Part print with two shaded views. Sizes in mm from the minimum x, y, z corner. Coordinates: 2 decimals unless noted, no trailing zeros. Loops run counter-clockwise (first coordinate to the right, second up) from the corner with the lowest first, then second, coordinate; pieces in that order, holes last. Notation, with made-up numbers: (28.5, 36.5) - (35.5, 36.5) arc R10 cw to (35.5, 52.5) - close; hole circle Ø3 at (12, 7.5). An arc over 180 degrees is marked (long way). Answer as CSV lines item,"result".
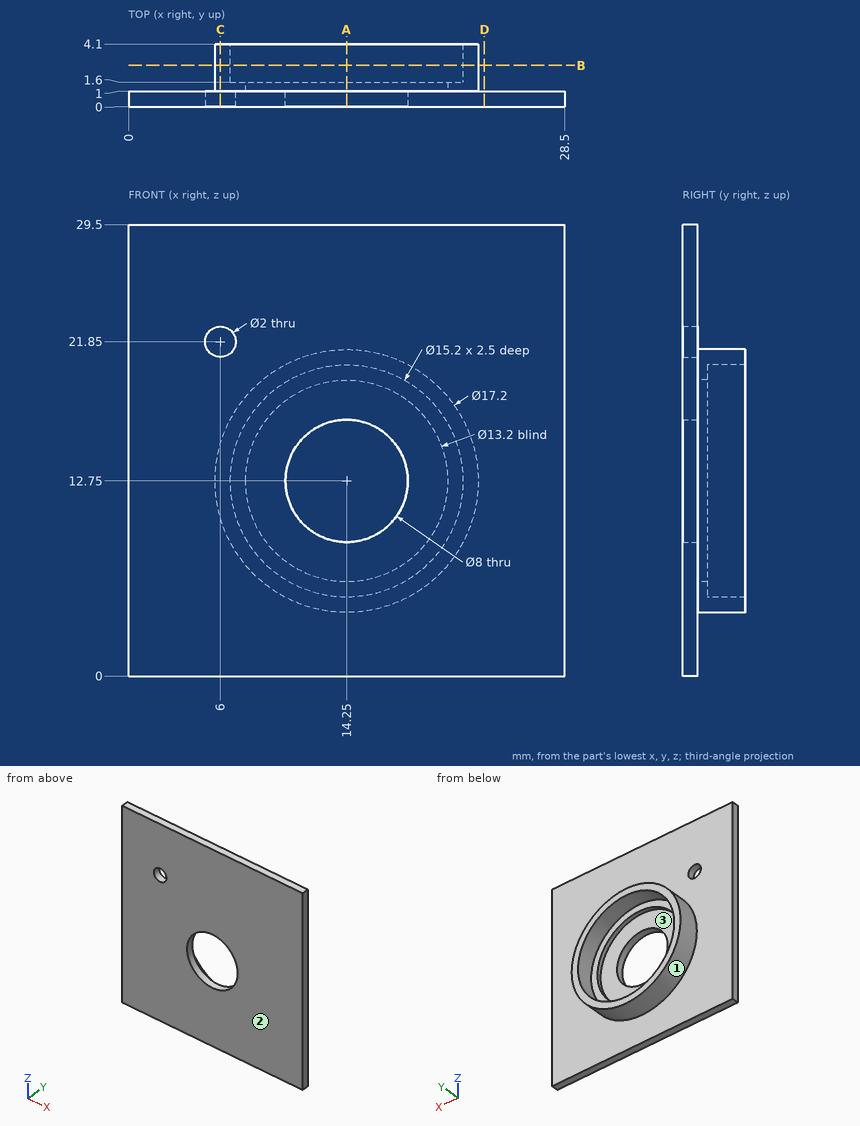
Q1. Saw through at C-C (x = 6). Give the cut face in (y, z).
Results:
outline,"(0, 0) - (1, 0) - (1, 10.32) - (4.1, 10.32) - (4.1, 15.18) - (1, 15.18) - (1, 20.85) - (0, 20.85) - close; (0, 22.85) - (1, 22.85) - (1, 29.5) - (0, 29.5) - close"
Q2. Wall check: L1, parallel to X at y = 0.7, z = 21.85; L2, parallel to Z at x = 14.25, y = 1.25; L3, parallel to Z at x = 6, y = 0.3. Give the ranges that are in metal, low to high.
Results:
L1,"x = 0 to 5, 7 to 28.5"
L2,"z = 4.15 to 6.15, 19.35 to 21.35"
L3,"z = 0 to 20.85, 22.85 to 29.5"
Q3. Two-plate mould, pull along Z, no slides. Class the marked faces 1, 2 and 3: released by +Z, released by -Z, zero draft, split by the parting line, or undercut.
Results:
face 1,"split by the parting line"
face 2,"zero draft"
face 3,"undercut"
Q4. Saw through at A-A (x = 14.25). Give the cut face in (y, z), then the cut area to 3 significant figures.
Results:
outline,"(0, 0) - (1, 0) - (1, 4.15) - (4.1, 4.15) - (4.1, 5.15) - (1.6, 5.15) - (1.6, 6.15) - (1, 6.15) - (1, 8.75) - (0, 8.75) - close; (0, 16.75) - (1, 16.75) - (1, 19.35) - (1.6, 19.35) - (1.6, 20.35) - (4.1, 20.35) - (4.1, 21.35) - (1, 21.35) - (1, 29.5) - (0, 29.5) - close"
area,"28.9 mm^2"
Q5. Flat gauge pins, fed straight in: pin 1 (8 mm diameter, centred on x = 6, z = 26, fed in from +Y); pin 2 (2 mm diameter, centred on y = 2.5, z = 19.5, fed in from +X); pin 3 (1.5 mm diameter, centred on y = 2.5, z = 6, fed in from -X). Where does each tip first touch, or does it go through?
Results:
pin 1,"stops at y = 1"
pin 2,"stops at x = 20.65"
pin 3,"stops at x = 8.09"
Q6. Saw through at D-D (x = 23.25). Give the cut face in (y, z), then the cut area to 3 significant figures.
Results:
outline,"(0, 0) - (1, 0) - (1, 29.5) - (0, 29.5) - close"
area,"29.5 mm^2"
Q7. Saw through at B-B (y = 2.7). Give the cut face in (x, z), then the cut area to 3 significant figures.
Results:
outline,"circle Ø17.2 at (14.25, 12.75); hole circle Ø15.2 at (14.25, 12.75)"
area,"50.9 mm^2"
